from build123d import *

# Parameters (mm, degrees)
SKETCH1_R           = 2
BOSS_EXTRUDE1_DEPTH = 40
SKETCH3_R           = 0.79375
CUT_EXTRUDE1_DEPTH  = 5
SKETCH4_R           = 0.79375
CUT_EXTRUDE2_DEPTH  = 5


with BuildPart() as part:
    # Sketch1 → Boss-Extrude1 (new, symmetric)
    with BuildSketch(Plane(origin=(0, 0, 0), x_dir=(1, 0, 0), z_dir=(0, 1, 0))):
        with Locations(Location((0, 0, 0), (0, 0, 270))):
            Circle(SKETCH1_R)
    extrude(amount=BOSS_EXTRUDE1_DEPTH, both=True)

    # Sketch3 → Cut-Extrude1 (cut, symmetric)
    with BuildSketch(Plane(origin=(0, 0, 0), x_dir=(0, 0, -1), z_dir=(1, 0, 0))):
        with Locations((0, 1)):
            Circle(SKETCH3_R)
        with Locations((0, 23)):
            Circle(SKETCH3_R)
    extrude(amount=CUT_EXTRUDE1_DEPTH, both=True, mode=Mode.SUBTRACT)

    # Sketch4 → Cut-Extrude2 (cut, symmetric)
    with BuildSketch(Plane(origin=(0, 0, 0), x_dir=(0, 0, -1), z_dir=(1, 0, 0))):
        with Locations((0, -16)):
            Circle(SKETCH4_R)
    extrude(amount=CUT_EXTRUDE2_DEPTH, both=True, mode=Mode.SUBTRACT)


solid = part.part
Can you work these out from the model? Positions are in its coordinate system, mm. Give positions to 0.01 mm unless a question says otherwise; leave off trailing zeros. Order: outer loops, then holes, each group sorted by start corner. A loop starts at its lowest first (then second) coordinate and runs counter-clockwise, first axis right, second up. Notation, with made-up numbers: M 47.5,-11 L 78.5,-11 A26 cw 78.5,25 Z; hole C -22,21.25 d6. An arc over 180 degrees is marked long. Use one line per item in the form item = value.
Item 1: If we section it at C-C, the plane y = -16: Write out the boundary of the cut face in (x, z).
Values follow:
outline = M -1.84,-0.79 A2 ccw 1.84,-0.79 Z; M -1.84,0.79 L 1.84,0.79 A2 ccw Z
Item 2: If we section it at B-B, the plane x = 0.65: Write out the boundary of the cut face in (y, z).
Values follow:
outline = M -40,-1.89 L 40,-1.89 L 40,1.89 L -40,1.89 Z; hole C -16,0 d1.59; hole C 1,0 d1.59; hole C 23,0 d1.59
Item 3: If we section it at A-A, the plane z = 0: Write out the boundary of the cut face in (x, y).
Values follow:
outline = M -2,-40 L 2,-40 L 2,-16.79 L -2,-16.79 Z; M -2,-15.21 L 2,-15.21 L 2,0.21 L -2,0.21 Z; M -2,1.79 L 2,1.79 L 2,22.21 L -2,22.21 Z; M -2,23.79 L 2,23.79 L 2,40 L -2,40 Z
Item 4: If we section it at D-D, the plane y = 13: Write out the boundary of the cut face in (x, z).
Values follow:
outline = C 0,0 d4
Item 5: Thinking about a two-plate mould opening in Z: for faces 1 (the flat face through (0, 40, 0)), 2 (the cylindrical face through (0.028, -15.331, -0.427)), 3 (the cylindrical face through (-0.766, 0.56, 1.847)), which applies, pulls with the +Z half, pulls with the -Z half, needs draft (parallel to the pull), parting line crosses it, or undercut?
Values follow:
face_1 = needs draft
face_2 = undercut
face_3 = parting line crosses it
Item 6: If I drill on line 1 along Y through (x, z) = (-1.5, 0); line 2 along Y through (x, z) = (-0.35, 0.5); line 3 along X through (y, z) = (18.5, 0.2), over which ranges is the centre line in solid material (lowest first)? Write a range as [from, to].
Values follow:
line_1 = [-40, -16.79], [-15.21, 0.21], [1.79, 22.21], [23.79, 40]
line_2 = [-40, -16.62], [-15.38, 0.38], [1.62, 22.38], [23.62, 40]
line_3 = [-1.99, 1.99]
